Read the model definition and answer for the solid it produces. Units are mm, in the model's axes. Face numbers are marked on the shaded views. A direction names the side the tool comes from. Give positions to 0.01 mm unless a question says otherwise; leave off trailing zeros. Write each loop counter-clockwise with the first axis right and the second up, starting at its lowest first coordinate (ties: lowest second). Pieces come first, ordered by that corner, then holes. Notation, with made-up numbers: (21, -26) -> (67, -26) arc R23 ccw to (67, 5) -> close; hole circle Ø5 at (-16, 1). An arc over 180 degrees is marked (long way). Put each result on its own line as item: value. Start each with the question number.
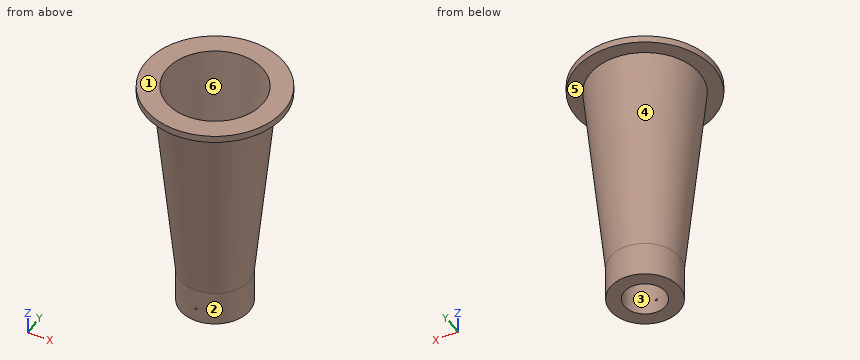
from build123d import *

# Parameters (mm, degrees)
SKETCH2_R          = 3
CUT_EXTRUDE1_DEPTH = 755.983443527


with BuildPart() as part:
    # Sketch1 → Revolve1 (revolve)
    with BuildSketch(Plane(origin=(0, 0, 0), x_dir=(1, 0, 0), z_dir=(0, 1, 0))):
        with BuildLine():
            Line((60, 700), (100, 700))
            Line((100, 700), (100, 600))
            Line((100, 600), (158.096747357, 20))
            Line((158.096747357, 20), (200, 20))
            Line((200, 20), (200, 0))
            Line((200, 0), (140, 0))
            Line((140, 0), (80.361922702, 595.387631955))
            ThreePointArc((80.361922702, 595.387631955), (78.741539447, 598.596831406), (75.386818985, 599.889291707))
            Line((75.386818985, 599.889291707), (60, 599.889291707))
            Line((60, 599.889291707), (60, 700))
        make_face()
    revolve(axis=Axis((0, 0, 396.040868455), (0, 0, -1)))

    # Sketch2 → Cut-Extrude1 (cut, through all)
    with BuildSketch(Plane(origin=(0, 0, 0), x_dir=(1, 0, 0), z_dir=(0, 1, 0))):
        with Locations(Location((0, 660, 0), (0, 0, 270))):
            Circle(SKETCH2_R)
    extrude(amount=-CUT_EXTRUDE1_DEPTH, mode=Mode.SUBTRACT)


solid = part.part
1) For the marked faces 1 and 2, determine the directions among +Z, -Z, +X, -X, +Y, -Y from which every point of the face is accessible in a straight line to the end or side of a thin tool.
2) For a pull along Y with two mould halves and no side action, classify the marked faces 3, 4, 5 and 6 as pulls with the +Y half, pulls with the -Y half, needs draft (parallel to the pull), parting line crosses it, or undercut.
3) Each of these flat-tipped pins is pushed along its axis until it touches: pin 1 Ø12 at (x, z) = (-130, -253.5) entering from +Y; pin 2 Ø5 at (y, z) = (-56.5, -587) entering from +X; pin 3 Ø5 at (y, z) = (-52, -385.5) entering from -X. Where does it stop, or does it pass through?
4) A cutting plane is placed at A-A on y = 0. Give the vertices of the cut face in (x, z), and give its area (3 significant figures).
5) A cutting plane is placed at C-C on z = -225. Give the vertices of the cut face in (x, y), and give its area (3 significant figures).
6) Straight lines are drawn through the part: line 1 (Z direction, x = 0, y = -72.5); line 2 (Y direction, x = 0, z = -621). For each, find the intervals that lie inside material, in ascending order. Write a range as [from, to].
7) A cutting plane is placed at B-B on z = -640.5. Give the vertices of the cut face in (x, y).
Results found:
1. face 1: +Z, +X, -X, +Y, -Y
1. face 2: -Z
2. face 3: undercut
2. face 4: parting line crosses it
2. face 5: needs draft
2. face 6: undercut
3. pin 1: stops at y = 52.72
3. pin 2: stops at x = 85.74
3. pin 3: stops at x = -110.98
4. outline: (-200, -20) -> (-158.1, -20) -> (-100, -600) -> (-100, -700) -> (-60, -700) -> (-60, -599.89) -> (-75.39, -599.89) arc R5 cw to (-80.36, -595.39) -> (-140, 0) -> (-200, 0) -> close; (60, -700) -> (100, -700) -> (100, -600) -> (158.1, -20) -> (200, -20) -> (200, 0) -> (140, 0) -> (80.36, -595.39) arc R5 cw to (75.39, -599.89) -> (60, -599.89) -> close
4. area: 33,800 mm²
5. outline: circle Ø275.13 at (0, 0); hole circle Ø234.92 at (0, 0)
5. area: 16,100 mm²
6. line 1: z = [-700, -663], [-657, -599.89]
6. line 2: y = [-100, -60], [60, 100]
7. outline: circle Ø200 at (0, 0); hole circle Ø120 at (0, 0)
